Geometry check sheet. Reference: the model listing, model coordinates, mm. A direction names the side the tool comes from. Coordinates: 2 decimals unless noted, no trailing zeros. Order: outer loops, then holes, each group sorted by start corner. A loop starts at its lowest first (then second) coordinate and runs counter-clockwise, first axis right, second up. Notation, with made-up numbers: (85, 74) - (118, 74) arc R35 ccw to (118, 106) - close; hole circle Ø9 at (19, 0.5). An arc over 180 degrees is marked (long way). Return JSON: item names as keys, results as strings. Group by question number.
Item 1: Draft check along Z on faces 1 (the flat face through (6, 26, 26.977)), 2 (the flat face through (-87.488, 26, -12)), 3 (the flat face through (6, 26, -53.023)), 4 (the flat face through (-14, 2, -14)). Enter one of: pulls with the +Z half, pulls with the -Z half, needs draft (parallel to the pull), parting line crosses it, or undercut.
Item 2: Gauge pin test, flat end, axial feed: pin 1 (0.9 mm diameter, centred on x = -84, z = -50.5, fed in from +Y). Record the tip position at first contact, or that the pin passes through.
Item 3: Tool access check on faces 5 (the flat face through (-15, 0, -14)), 6 (the flat face through (6, 27, 24.977)). Record the directions out of +Z, -Z, +X, -X, +Y, -Y that give a thin tool (end or side, any length) a straight path to the whole face; none if there is none.
Item 4: Section check D-D on z = 11.5. Enter the section's corners in (x, y), then the cut area to 3 significant figures.
Item 5: Scan lines: probe 1 along Z at (x, y) = (-69, 37); probe 2 along X at (y, z) = (32.5, 8); probe 3 along Y at (x, z) = (-62, -18). Record each from-to range of solid material in increasing order.
Item 6: Section check A-A on x = -46. Enter the section's corners in (y, z), then the cut area to 3 significant figures.
Item 7: Section check B-B on z = -17. Enter the section's corners in (x, y), then the cut area to 3 significant figures.
Item 8: Section check C-C on y = 21. Enter the section's corners in (x, z), then the cut area to 3 significant figures.
from build123d import *

# Parameters (mm, degrees)
SKETCH1_W           = 190
SKETCH1_H           = 80
BOSS_EXTRUDE1_DEPTH = 2
SKETCH2_W           = 190
SKETCH2_H           = 80
SKETCH2_R           = 1.5
SKETCH2_R_2         = 1.55
BOSS_EXTRUDE2_DEPTH = 50
SKETCH3_R           = 1.2
SKETCH3_R_2         = 1.55
SKETCH3_W           = 34.1
SKETCH3_H           = 23.1
CUT_EXTRUDE1_DEPTH  = 127.586332253


with BuildPart() as part:
    # Sketch1 → Boss-Extrude1 (new body)
    with BuildSketch(Plane(origin=(0, 0, 0), x_dir=(1, 0, 0), z_dir=(0, 1, 0))):
        with Locations((7.511627907, 13.023255814)):
            Rectangle(SKETCH1_W, SKETCH1_H)
    extrude(amount=BOSS_EXTRUDE1_DEPTH)

    # Sketch2 → Boss-Extrude2 (add)
    with BuildSketch(Plane(origin=(0, 2, 0), x_dir=(1, 0, 0), z_dir=(0, 1, 0))):
        with Locations((7.511627907, 13.023255814)):
            Rectangle(SKETCH2_W, SKETCH2_H)
        with Locations(Location((-84.488372093, -23.976744186, 0), (0, 0, 270))):
            Circle(SKETCH2_R, mode=Mode.SUBTRACT)
        with Locations(Location((99.511627907, -23.976744186, 0), (0, 0, 270))):
            Circle(SKETCH2_R, mode=Mode.SUBTRACT)
        with Locations(Location((99.511627907, 50.023255814, 0), (0, 0, 270))):
            Circle(SKETCH2_R_2, mode=Mode.SUBTRACT)
        with Locations(Location((-84.488372093, 50.023255814, 0), (0, 0, 270))):
            Circle(SKETCH2_R_2, mode=Mode.SUBTRACT)
        with BuildLine():
            Line((-81.488372093, -23.976744186), (-81.488372093, -24.976744186))
            Line((-81.488372093, -24.976744186), (96.683200782, -24.976744186))
            ThreePointArc((96.683200782, -24.976744186), (97.062138164, -22.244693378), (99.511627907, -20.976744186))
            Line((99.511627907, -20.976744186), (100.511627907, -20.976744186))
            Line((100.511627907, -20.976744186), (100.511627907, 47.023255814))
            Line((100.511627907, 47.023255814), (99.511627907, 47.023255814))
            ThreePointArc((99.511627907, 47.023255814), (97.390307563, 47.90193547), (96.511627907, 50.023255814))
            Line((96.511627907, 50.023255814), (96.511627907, 51.023255814))
            Line((96.511627907, 51.023255814), (-81.488372093, 51.023255814))
            Line((-81.488372093, 51.023255814), (-81.488372093, 50.023255814))
            ThreePointArc((-81.488372093, 50.023255814), (-82.367051749, 47.90193547), (-84.488372093, 47.023255814))
            Line((-84.488372093, 47.023255814), (-85.488372093, 47.023255814))
            Line((-85.488372093, 47.023255814), (-85.488372093, -20.976744186))
            Line((-85.488372093, -20.976744186), (-84.488372093, -20.976744186))
            ThreePointArc((-84.488372093, -20.976744186), (-82.367051749, -21.855423842), (-81.488372093, -23.976744186))
        make_face(mode=Mode.SUBTRACT)
    extrude(amount=BOSS_EXTRUDE2_DEPTH)

    # Sketch3 → Cut-Extrude1 (cut, through all)
    with BuildSketch(Plane.XZ):
        with Locations(Location((25.111627907, 16.326744186, 0), (0, 0, 270))):
            Circle(SKETCH3_R)
        with Locations(Location((84.911627907, 16.326744186, 0), (0, 0, 270))):
            Circle(SKETCH3_R)
        with Locations(Location((25.111627907, -42.373255814, 0), (0, 0, 270))):
            Circle(SKETCH3_R)
        with Locations(Location((84.911627907, -42.373255814, 0), (0, 0, 270))):
            Circle(SKETCH3_R)
        with Locations(Location((-55.338372093, 1.776744186, 0), (0, 0, 270))):
            Circle(SKETCH3_R_2)
        with Locations(Location((-24.138372093, 1.776744186, 0), (0, 0, 270))):
            Circle(SKETCH3_R_2)
        with Locations(Location((-55.338372093, -27.523255814, 0), (0, 0, 270))):
            Circle(SKETCH3_R_2)
        with Locations(Location((-24.138372093, -27.523255814, 0), (0, 0, 270))):
            Circle(SKETCH3_R_2)
        with BuildLine():
            Line((26.961627907, 15.526744186), (83.061627907, 15.526744186))
            ThreePointArc((83.061627907, 15.526744186), (84.475841469, 14.940957748), (85.061627907, 13.526744186))
            Line((85.061627907, 13.526744186), (85.061627907, -39.573255814))
            ThreePointArc((85.061627907, -39.573255814), (84.475841469, -40.987469376), (83.061627907, -41.573255814))
            Line((83.061627907, -41.573255814), (26.961627907, -41.573255814))
            ThreePointArc((26.961627907, -41.573255814), (25.547414345, -40.987469376), (24.961627907, -39.573255814))
            Line((24.961627907, -39.573255814), (24.961627907, 13.526744186))
            ThreePointArc((24.961627907, 13.526744186), (25.547414345, 14.940957748), (26.961627907, 15.526744186))
        make_face()
        with Locations((-39.738372093, -13.043255814)):
            Rectangle(SKETCH3_W, SKETCH3_H)
    extrude(amount=-CUT_EXTRUDE1_DEPTH, mode=Mode.SUBTRACT)


solid = part.part
Computed:
{
 "1": {"face 1": "pulls with the +Z half", "face 2": "needs draft", "face 3": "pulls with the -Z half", "face 4": "undercut"},
 "2": {"pin 1": "stops at y = 2"},
 "3": {"face 5": "+Z, -Z, +X, -X, -Y", "face 6": "+Y"},
 "4": {"outline": "(-87.49, 0) - (24.96, 0) - (24.96, 2) - (-85.49, 2) - (-85.49, 52) - (-87.49, 52) - close; (85.06, 0) - (102.51, 0) - (102.51, 52) - (100.51, 52) - (100.51, 2) - (85.06, 2) - close", "area": "460 mm²"},
 "5": {"probe 1": "z = -53.02 to -51.02, 24.98 to 26.98", "probe 2": "x = -87.49 to -85.49, 100.51 to 102.51", "probe 3": "y = 0 to 2"},
 "6": {"outline": "(0, -53.02) - (52, -53.02) - (52, -51.02) - (2, -51.02) - (2, -24.59) - (0, -24.59) - close; (0, -1.49) - (2, -1.49) - (2, 24.98) - (52, 24.98) - (52, 26.98) - (0, 26.98) - close", "area": "314 mm²"},
 "7": {"outline": "(-87.49, 0) - (-56.79, 0) - (-56.79, 2) - (-85.49, 2) - (-85.49, 52) - (-87.49, 52) - close; (-22.69, 0) - (24.96, 0) - (24.96, 2) - (-22.69, 2) - close; (85.06, 0) - (102.51, 0) - (102.51, 52) - (100.51, 52) - (100.51, 2) - (85.06, 2) - close", "area": "392 mm²"},
 "8": {"outline": "(-87.49, -53.02) - (102.51, -53.02) - (102.51, 26.98) - (-87.49, 26.98) - close; hole circle Ø3.1 at (-84.49, -50.02); hole circle Ø3 at (-84.49, 23.98); hole (-85.49, -47.02) - (-84.49, -47.02) arc R3 cw to (-81.49, -50.02) - (-81.49, -51.02) - (96.51, -51.02) - (96.51, -50.02) arc R3 cw to (99.51, -47.02) - (100.51, -47.02) - (100.51, 20.98) - (99.51, 20.98) arc R3 cw to (96.68, 24.98) - (-81.49, 24.98) - (-81.49, 23.98) arc R3 cw to (-84.49, 20.98) - (-85.49, 20.98) - close; hole circle Ø3.1 at (99.51, -50.02); hole circle Ø3 at (99.51, 23.98)", "area": "1,090 mm²"}
}
